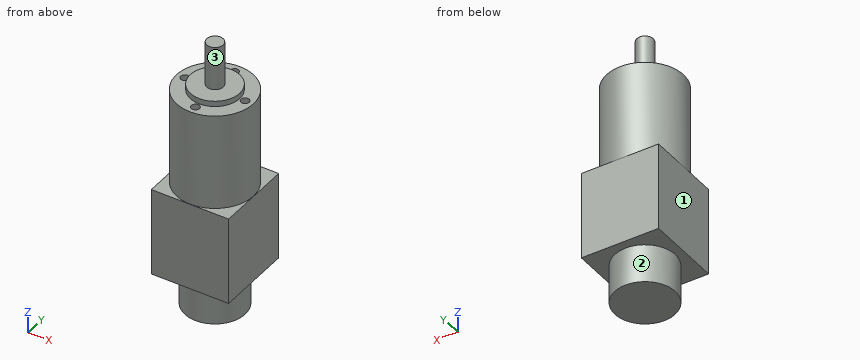
```python
from build123d import *

# Parameters (mm, degrees)
SKETCH_W     = 28.2
SKETCH_H     = 28.2
PAD_DEPTH    = 32
SKETCH002_R  = 14
PAD001_DEPTH = 35
SKETCH003_R  = 9
PAD002_DEPTH = 2
SKETCH004_R  = 3
PAD003_DEPTH = 16
SKETCH005_R  = 11
PAD004_DEPTH = 14
SKETCH006_R  = 1.5
POCKET_DEPTH = 5


with BuildPart() as part:
    # Sketch → Pad (new body)
    with BuildSketch(Plane.XY):
        Rectangle(SKETCH_W, SKETCH_H)
    extrude(amount=PAD_DEPTH)

    # Sketch002 → Pad001 (join)
    with BuildSketch(Plane.XY.offset(32)):
        Circle(SKETCH002_R)
    extrude(amount=PAD001_DEPTH)

    # Sketch003 → Pad002 (join)
    with BuildSketch(Plane.XY.offset(67)):
        Circle(SKETCH003_R)
    extrude(amount=PAD002_DEPTH)

    # Sketch004 → Pad003 (join)
    with BuildSketch(Plane.XY.offset(69)):
        Circle(SKETCH004_R)
    extrude(amount=PAD003_DEPTH)

    # Sketch005 → Pad004 (join)
    with BuildSketch(Plane.XY):
        Circle(SKETCH005_R)
    extrude(amount=-PAD004_DEPTH)

    # Sketch006 → Pocket (cut)
    with BuildSketch(Plane(origin=(0, 0, 67), x_dir=(0.707107, 0.707107, 0), z_dir=(0, 0, 1))):
        with Locations((-7.778175, 7.778175)):
            Circle(SKETCH006_R)
        with Locations((7.778175, 7.778175)):
            Circle(SKETCH006_R)
        with Locations((7.778175, -7.778175)):
            Circle(SKETCH006_R)
        with Locations((-7.778175, -7.778175)):
            Circle(SKETCH006_R)
    extrude(amount=-POCKET_DEPTH, mode=Mode.SUBTRACT)


solid = part.part
```
Geometry: final body of the model. Coordinates: model frame, mm. Face numbers are marked on the shaded views. A direction names the side the tool comes from. Round coordinates to 2 decimals unless told otherwise and drop trailing zeros. Loops run counter-clockwise (first coordinate to the right, second up) from the corner with the lowest first, then second, coordinate; pieces in that order, holes last. Notation, with made-up numbers: (62.5, 17) -> (103.5, 17) arc R27 cw to (103.5, 39) -> close; hole circle Ø7 at (-1, 67). An arc over 180 degrees is marked (long way). Write each question's results on one line, items separated by ' | '.
Item 1: Line query: probe 1 along Z at (x, y) = (2, -11.5); probe 2 along Z at (x, y) = (1.5, -5.5); probe 3 along X at (y, z) = (11, 64.65). Output: solid intervals per line, ascending. Write a range as [from, to].
Answers below:
probe 1: z = [0, 67] | probe 2: z = [-14, 69] | probe 3: x = [-8.66, -1.5], [1.5, 8.66]
Item 2: Cut plane C-C on z = 52. Return the cut outline in (x, y).
Answers below:
outline: circle Ø28 at (0, 0)
Item 3: Set-up query: the marked faces 1, 2 and 3. Return all of +Z, -Z, +X, -X, +Y, -Y with unobstructed straight access to the full face (end or side cutting, diameter ignored); none if empty.
Answers below:
face 1: +Z, -Z, -X, +Y, -Y | face 2: -Z | face 3: +Z
Item 4: Pin query (flat end, axial travel): pin 1 Ø8 at (x, y) = (11.5, -9.5) entering from +Z; pin 2 Ø2.5 at (x, y) = (0, 11) entering from +Z; pin 3 Ø12 at (x, z) = (10, 59.5) entering from -Y. Return the tip coordinate at first contact, or that it passes through.
Answers below:
pin 1: stops at z = 67 | pin 2: stops at z = 62 | pin 3: stops at y = -13.42
Item 5: Cut plane D-D on y = -7.75. Return the cut outline in (x, z).
Answers below:
outline: (-14.1, 0) -> (-7.81, 0) -> (-7.81, -14) -> (7.81, -14) -> (7.81, 0) -> (14.1, 0) -> (14.1, 32) -> (11.66, 32) -> (11.66, 67) -> (4.58, 67) -> (4.58, 69) -> (-4.58, 69) -> (-4.58, 67) -> (-11.66, 67) -> (-11.66, 32) -> (-14.1, 32) -> close
Item 6: Cut plane A-A on x = 0. Return the cut outline in (y, z).
Answers below:
outline: (-14.1, 0) -> (-11, 0) -> (-11, -14) -> (11, -14) -> (11, 0) -> (14.1, 0) -> (14.1, 32) -> (14, 32) -> (14, 67) -> (12.5, 67) -> (12.5, 62) -> (9.5, 62) -> (9.5, 67) -> (9, 67) -> (9, 69) -> (3, 69) -> (3, 85) -> (-3, 85) -> (-3, 69) -> (-9, 69) -> (-9, 67) -> (-9.5, 67) -> (-9.5, 62) -> (-12.5, 62) -> (-12.5, 67) -> (-14, 67) -> (-14, 32) -> (-14.1, 32) -> close
